For this review, take the finished solid that the model builds, in its own axes (mm). A direction names the side the tool comes from. Give positions to 0.01 mm unless a question says otherwise; leave off trailing zeros. Loops run counter-clockwise (first coordinate to the right, second up) from the corner with the lowest first, then second, coordinate; pieces in that order, holes last. Notation, with made-up numbers: (-29.75, 31.25) -> (10.25, 31.25) arc R32 cw to (10.25, 70.25) -> close; hole circle Ø5 at (45.25, -2). An arc over 180 degrees is marked (long way). Answer as CSV lines item,"result". Start each with the question number.
Item 1: Add section C-C on x = 19. State the section outline as (y, z) points, plus the area to 3 significant figures.
Item 2: The part is to be moulded in two halves that separate along Z. For faces 1 (the face through (-17.542, -18.884, 6.826)), 2 (the face through (17.997, 0.631, 9.86)), 3 (the face through (-9, 34, 10)), say which applies: +Z half, -Z half, draft (parallel to the pull), parting line (faces both ways), or undercut.
Item 3: Machinability: for faces 4 (the face through (13.9, -23.88, 10.14)), 5 (the face through (-23.035, -15.031, 8.452)), 6 (the face through (-20.5, -18, 12)), 7 (the face through (-9.094, 36.132, 15.07)), which of the approach directions +Z, -Z, +X, -X, +Y, -Y give a long, thin tool a straight path to every point of the face, cutting with its end or side? Answer none if there is none.
Item 4: Add section B-B on y = 0. State the section outline as (x, z) points, plus the area to 4 significant figures.
Item 5: Add section A-A on y = -16.45. State the section outline as (x, z) points.
Item 6: For L1, parallel to Y at x = -23.5, z = 10; L2, parallel to X at y = -1, z = 3.5; L3, parallel to X at y = 16, z = 18, list the stretches that pass through material, from the lowest coordinate up. Write a range as from..to.
Item 7: Add section D-D on y = 34.05. State the section outline as (x, z) points, plus the area to 3 significant figures.
Item 8: Clearance check with flat-ended pins moving along their axes: P1, Ø8, axis at y = 27, z = 11, coming from the +X side; P2, Ø2.5, axis at y = 18, z = 9, coming from the +X side; P3, Ø1.3, axis at x = -19.5, y = -25.5, coming from the +Z side. State where each tip first meets the part, or that it passes through.
```python
from build123d import *

# Parameters (mm, degrees)
SKETCH1_W           = 29
SKETCH1_H           = 48.9
BOSS_EXTRUDE1_DEPTH = 20
SKETCH2_R           = 2.1
CUT_EXTRUDE1_DEPTH  = 52.909079167
FILLET1_R           = 2
FILLET2_R           = 10
CHAMFER1_SIZE       = 1
CUT_EXTRUDE2_REACH  = 70.156
SKETCH3_R           = 2.1
CUT_EXTRUDE3_REACH  = 66.5
SKETCH4_R           = 4
SKETCH5_R           = 2.1
CUT_EXTRUDE4_DEPTH  = 10


with BuildPart() as part:
    # Sketch1 → Boss-Extrude1 (new body)
    with BuildSketch(Plane.XY):
        Polygon((-25.5, 40.55), (5.5, 40.55), (25.5, 20.55), (25.5, -31.45), (-25.5, -31.45), align=None)
        Rectangle(SKETCH1_W, SKETCH1_H, mode=Mode.SUBTRACT)
    extrude(amount=BOSS_EXTRUDE1_DEPTH)

    # Sketch2 → Cut-Extrude1 (cut, through all)
    with BuildSketch(Plane(origin=(0, 0, 0), x_dir=(-1, 0, 0), z_dir=(0, 0, -1))):
        with Locations((-20, 0)):
            Circle(SKETCH2_R)
        with Locations((20, 0)):
            Circle(SKETCH2_R)
    extrude(amount=-CUT_EXTRUDE1_DEPTH, mode=Mode.SUBTRACT)

    # Fillet1
    fillet1_edges = [part.edges().sort_by_distance(p)[0] for p in [
        (14.5, -24.45, 10),
        (14.5, 24.45, 10),
        (-14.5, 24.45, 10),
        (-14.5, -24.45, 10),
    ]]
    fillet(fillet1_edges, radius=FILLET1_R)

    # Fillet2
    fillet2_edges = [part.edges().sort_by_distance(p)[0] for p in [
        (5.5, 40.55, 10),
        (25.5, 20.55, 10),
    ]]
    fillet(fillet2_edges, radius=FILLET2_R)

    # Chamfer1
    chamfer1_edges = [part.edges().sort_by_distance(p)[0] for p in [
        (25.5, -7.521067812, 0),
        (15.5, 30.55, 0),
        (-12.071067812, 40.55, 0),
        (5.1846987, 39.788795325, 0),
        (24.738795325, 20.2346987, 0),
    ]]
    chamfer(chamfer1_edges, length=CHAMFER1_SIZE)

    # Sketch3 → Cut-Extrude2 (cut, up to next)
    with BuildSketch(Plane.ZY.offset(25.5), mode=Mode.PRIVATE) as cut_extrude2_sk1:
        with Locations((10, 16.55)):
            Circle(SKETCH3_R)
    cut_extrude2_tool1 = extrude(cut_extrude2_sk1.sketch, amount=-CUT_EXTRUDE2_REACH, mode=Mode.PRIVATE) & part.part
    # Sketch3 → Cut-Extrude2 (cut, up to next)
    with BuildSketch(Plane.ZY.offset(25.5), mode=Mode.PRIVATE) as cut_extrude2_sk2:
        with Locations((10, -16.45)):
            Circle(SKETCH3_R)
    cut_extrude2_tool2 = extrude(cut_extrude2_sk2.sketch, amount=-CUT_EXTRUDE2_REACH, mode=Mode.PRIVATE) & part.part
    add(cut_extrude2_tool1.solids().sort_by_distance((-25.5, 16.55, 10))[0], mode=Mode.SUBTRACT)
    add(cut_extrude2_tool2.solids().sort_by_distance((-25.5, -16.45, 10))[0], mode=Mode.SUBTRACT)

    # Sketch4 → Cut-Extrude3 (cut, up to next)
    with BuildSketch(Plane.ZY.offset(20.5), mode=Mode.PRIVATE) as cut_extrude3_sk1:
        with Locations((10, 16.55)):
            Circle(SKETCH4_R)
    cut_extrude3_tool1 = extrude(cut_extrude3_sk1.sketch, amount=-CUT_EXTRUDE3_REACH, mode=Mode.PRIVATE) & part.part
    # Sketch4 → Cut-Extrude3 (cut, up to next)
    with BuildSketch(Plane.ZY.offset(20.5), mode=Mode.PRIVATE) as cut_extrude3_sk2:
        with Locations((10, -16.45)):
            Circle(SKETCH4_R)
    cut_extrude3_tool2 = extrude(cut_extrude3_sk2.sketch, amount=-CUT_EXTRUDE3_REACH, mode=Mode.PRIVATE) & part.part
    add(cut_extrude3_tool1.solids().sort_by_distance((-20.5, 16.55, 10))[0], mode=Mode.SUBTRACT)
    add(cut_extrude3_tool2.solids().sort_by_distance((-20.5, -16.45, 10))[0], mode=Mode.SUBTRACT)

    # Sketch5 → Cut-Extrude4 (cut)
    with BuildSketch(Plane.XY.offset(20)):
        with Locations((19, -24.95)):
            Circle(SKETCH5_R)
        with Locations((-8.821067812, 34.05)):
            Circle(SKETCH5_R)
        with Locations((-19, -24.95)):
            Circle(SKETCH5_R)
    extrude(amount=-CUT_EXTRUDE4_DEPTH, mode=Mode.SUBTRACT)


solid = part.part
```
Computed values:
1,outline,"(-31.45, 0) -> (-1.85, 0) -> (-1.85, 20) -> (-22.85, 20) -> (-22.85, 10) -> (-27.05, 10) -> (-27.05, 20) -> (-31.45, 20) -> close; (1.85, 0) -> (25.64, 0) -> (27.05, 1) -> (27.05, 20) -> (1.85, 20) -> close"
1,area,"1,050 mm²"
2,face 1,"undercut"
2,face 2,"draft"
2,face 3,"+Z half"
3,face 4,"+Z, -Z"
3,face 5,"-X"
3,face 6,"none"
3,face 7,"+Z"
4,outline,"(-25.5, 0) -> (-22.1, 0) -> (-22.1, 20) -> (-25.5, 20) -> close; (-17.9, 0) -> (-14.5, 0) -> (-14.5, 20) -> (-17.9, 20) -> close; (14.5, 0) -> (17.9, 0) -> (17.9, 20) -> (14.5, 20) -> close; (22.1, 0) -> (24.5, 0) -> (25.5, 1) -> (25.5, 20) -> (22.1, 20) -> close"
4,area,"271.5 mm²"
5,outline,"(-25.5, 0) -> (-14.5, 0) -> (-14.5, 6) -> (-20.5, 6) -> (-20.5, 7.9) -> (-25.5, 7.9) -> close; (-25.5, 12.1) -> (-20.5, 12.1) -> (-20.5, 14) -> (-14.5, 14) -> (-14.5, 20) -> (-25.5, 20) -> close; (14.5, 0) -> (24.5, 0) -> (25.5, 1) -> (25.5, 20) -> (14.5, 20) -> close"
6,L1,"-31.45..-18.55, -14.35..14.45, 18.65..40.55"
6,L2,"-25.5..-21.85, -18.15..-14.5, 14.5..18.15, 21.85..25.5"
6,L3,"-25.5..-14.5, 14.5..25.5"
7,outline,"(-25.5, 0) -> (10.59, 0) -> (12, 1) -> (12, 20) -> (-6.72, 20) -> (-6.72, 10) -> (-10.92, 10) -> (-10.92, 20) -> (-25.5, 20) -> close"
7,area,"707 mm²"
8,P1,"x = 23.02"
8,P2,"x = 25.49"
8,P3,"z = 10"
